```python
from build123d import *

# Parameters (mm, degrees)
ESTRUSIONE_ESTRUSIONE1_DEPTH = 18


with BuildPart() as part:
    # Schizzo1 → Estrusione-Estrusione1 (new body)
    with BuildSketch(Plane.XY):
        with BuildLine():
            Line((-152, 250), (-152, 232))
            ThreePointArc((-152, 232), (-155.175, 228.825), (-158.35, 232))
            Line((-158.35, 232), (-232, 232))
            Line((-232, 232), (-232, 158.35))
            ThreePointArc((-232, 158.35), (-228.825, 155.175), (-232, 152))
            Line((-232, 152), (-250, 152))
            Line((-250, 152), (-250, 102))
            Line((-250, 102), (-232, 102))
            ThreePointArc((-232, 102), (-228.825, 98.825), (-232, 95.65))
            Line((-232, 95.65), (-232, 31.35))
            ThreePointArc((-232, 31.35), (-228.825, 28.175), (-232, 25))
            Line((-232, 25), (-250, 25))
            Line((-250, 25), (-250, -25))
            Line((-250, -25), (-232, -25))
            ThreePointArc((-232, -25), (-228.825, -28.175), (-232, -31.35))
            Line((-232, -31.35), (-232, -95.65))
            ThreePointArc((-232, -95.65), (-228.825, -98.825), (-232, -102))
            Line((-232, -102), (-250, -102))
            Line((-250, -102), (-250, -152))
            Line((-250, -152), (-232, -152))
            ThreePointArc((-232, -152), (-228.825, -155.175), (-232, -158.35))
            Line((-232, -158.35), (-232, -232))
            Line((-232, -232), (-158.35, -232))
            ThreePointArc((-158.35, -232), (-155.175, -228.825), (-152, -232))
            Line((-152, -232), (-152, -250))
            Line((-152, -250), (-102, -250))
            Line((-102, -250), (-102, -232))
            ThreePointArc((-102, -232), (-98.825, -228.825), (-95.65, -232))
            Line((-95.65, -232), (-31.35, -232))
            ThreePointArc((-31.35, -232), (-28.175, -228.825), (-25, -232))
            Line((-25, -232), (-25, -250))
            Line((-25, -250), (25, -250))
            Line((25, -250), (25, -232))
            ThreePointArc((25, -232), (28.175, -228.825), (31.35, -232))
            Line((31.35, -232), (95.65, -232))
            ThreePointArc((95.65, -232), (98.825, -228.825), (102, -232))
            Line((102, -232), (102, -250))
            Line((102, -250), (152, -250))
            Line((152, -250), (152, -232))
            ThreePointArc((152, -232), (155.175, -228.825), (158.35, -232))
            Line((158.35, -232), (232, -232))
            Line((232, -232), (232, -158.35))
            ThreePointArc((232, -158.35), (228.825, -155.175), (232, -152))
            Line((232, -152), (250, -152))
            Line((250, -152), (250, -102))
            Line((250, -102), (232, -102))
            ThreePointArc((232, -102), (228.825, -98.825), (232, -95.65))
            Line((232, -95.65), (232, -31.35))
            ThreePointArc((232, -31.35), (228.825, -28.175), (232, -25))
            Line((232, -25), (250, -25))
            Line((250, -25), (250, 25))
            Line((250, 25), (232, 25))
            ThreePointArc((232, 25), (228.825, 28.175), (232, 31.35))
            Line((232, 31.35), (232, 95.65))
            ThreePointArc((232, 95.65), (228.825, 98.825), (232, 102))
            Line((232, 102), (250, 102))
            Line((250, 102), (250, 152))
            Line((250, 152), (232, 152))
            ThreePointArc((232, 152), (228.825, 155.175), (232, 158.35))
            Line((232, 158.35), (232, 232))
            Line((232, 232), (158.35, 232))
            ThreePointArc((158.35, 232), (155.175, 228.825), (152, 232))
            Line((152, 232), (152, 250))
            Line((152, 250), (102, 250))
            Line((102, 250), (102, 232))
            ThreePointArc((102, 232), (98.825, 228.825), (95.65, 232))
            Line((95.65, 232), (31.35, 232))
            ThreePointArc((31.35, 232), (28.175, 228.825), (25, 232))
            Line((25, 232), (25, 250))
            Line((25, 250), (-25, 250))
            Line((-25, 250), (-25, 232))
            ThreePointArc((-25, 232), (-28.175, 228.825), (-31.35, 232))
            Line((-31.35, 232), (-95.65, 232))
            ThreePointArc((-95.65, 232), (-98.825, 228.825), (-102, 232))
            Line((-102, 232), (-102, 250))
            Line((-102, 250), (-152, 250))
        make_face()
        with BuildLine():
            Line((134.65, 95.646711769), (134.65, 116.646711769))
            Line((134.65, 116.646711769), (155.65, 116.646711769))
            ThreePointArc((155.65, 116.646711769), (158.825, 119.821711769), (155.65, 122.996711769))
            Line((155.65, 122.996711769), (155.65, 128.296711769))
            ThreePointArc((155.65, 128.296711769), (158.825, 131.471711769), (155.65, 134.646711769))
            Line((155.65, 134.646711769), (134.65, 134.646711769))
            Line((134.65, 134.646711769), (134.65, 155.646711769))
            ThreePointArc((134.65, 155.646711769), (131.475, 158.821711769), (128.3, 155.646711769))
            Line((128.3, 155.646711769), (123, 155.646711769))
            ThreePointArc((123, 155.646711769), (119.825, 158.821711769), (116.65, 155.646711769))
            Line((116.65, 155.646711769), (116.65, 134.646711769))
            Line((116.65, 134.646711769), (95.65, 134.646711769))
            ThreePointArc((95.65, 134.646711769), (92.475, 131.471711769), (95.65, 128.296711769))
            Line((95.65, 128.296711769), (95.65, 122.996711769))
            ThreePointArc((95.65, 122.996711769), (92.475, 119.821711769), (95.65, 116.646711769))
            Line((95.65, 116.646711769), (116.65, 116.646711769))
            Line((116.65, 116.646711769), (116.65, 95.646711769))
            ThreePointArc((116.65, 95.646711769), (119.825, 92.471711769), (123, 95.646711769))
            Line((123, 95.646711769), (128.3, 95.646711769))
            ThreePointArc((128.3, 95.646711769), (131.475, 92.471711769), (134.65, 95.646711769))
        make_face(mode=Mode.SUBTRACT)
    extrude(amount=ESTRUSIONE_ESTRUSIONE1_DEPTH)


solid = part.part
```
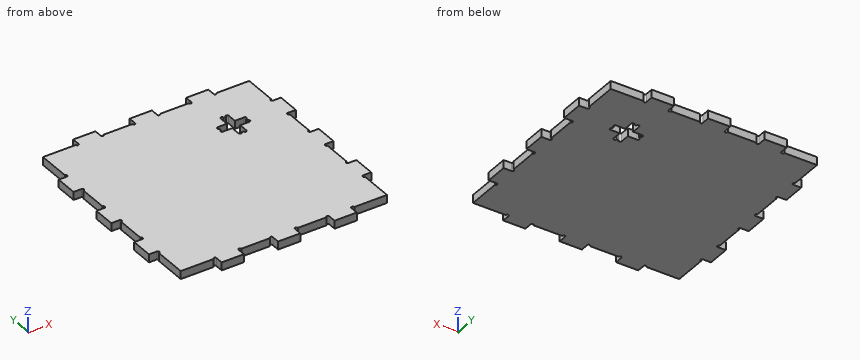
CAD build for the part. Positions are in the model's coordinates, mm. Coordinates: 2 decimals unless noted, no trailing zeros. Order: outer loops, then holes, each group sorted by start corner. A loop starts at its lowest first (then second) coordinate and runs counter-clockwise, first axis right, second up. Notation, with made-up numbers: (-7, 1.25) - (34, 1.25) arc R15 ccw to (34, 26.25) - close; hole circle Ø2 at (72.5, 71.25). An arc over 180 degrees is marked (long way). Answer in a Markdown table with one row per item.
1. Slice it at A-A, the plane y = 210. List the corners of the cut face in (x, z), then the cut area to 3 significant figures.
Answer:
| item | result |
|---|---|
| outline | (-232, 0) - (232, 0) - (232, 18) - (-232, 18) - close |
| area | 8,350 mm² |
2. Drill centre lines: L1, parallel to X at y = 105, z = 14.25; L2, parallel to X at y = 33, z = 12.5. Where is each one in solid material? Low to high. Write a range as from..to.
Answer:
| item | result |
|---|---|
| L1 | -250..116.65, 134.65..250 |
| L2 | -232..232 |
3. Flat gauge pins, fed straight in: P1, Ø1, axis at y = 195, z = 3.5, coming from the -X side; P2, Ø5.5, axis at x = 237.5, z = 9, coming from the -Y side; P3, Ø9, axis at x = -204.5, z = 9.5, coming from the -Y side. Where does each tip first touch, or does it go through?
Answer:
| item | result |
|---|---|
| P1 | x = -232 |
| P2 | y = -152 |
| P3 | y = -232 |
